Here's how the part is built. I have some questions about the finished solid (model axes, mm). Round coordinates to 2 decimals unless told otherwise and drop trailing zeros. Loops run counter-clockwise (first coordinate to the right, second up) from the corner with the lowest first, then second, coordinate; pieces in that order, holes last. Notation, with made-up numbers: M 85.5,-7.5 L 116.5,-7.5 A9 cw 116.5,9.5 Z; hole C 35.25,14 d6. An arc over 180 degrees is marked long. Use a Markdown table: item, result.
from build123d import *

# Parameters (mm, degrees)
F1_DEPTH = 25.4


# Not quite as in the source:
# - a feature names something its author has since deleted; it is built from what else it names


with BuildPart() as f1:
    # F0 (on Front) → F1 (new body)
    with BuildSketch(Plane.XZ):
        with BuildLine():
            Line((-23.1970027089, 51.8983751535), (-44.2315712571, 16.1199513823))
            Line((-44.2315712571, 16.1199513823), (-28.70137633, 16.1199513823))
            ThreePointArc((-28.70137633, 16.1199513823), (-16.1199513823, 22.0364309456), (-3.5385264346, 16.1199513823))
            Line((-3.5385264346, 16.1199513823), (44.2315712571, 16.1199513823))
            Line((44.2315712571, 16.1199513823), (-23.1970027089, 51.8983751535))
        make_face()
        with BuildLine():
            Line((-28.70137633, 16.1199513823), (-44.2315712571, 16.1199513823))
            Line((-44.2315712571, 16.1199513823), (-44.2315712571, -16.1199513823))
            Line((-44.2315712571, -16.1199513823), (44.2315712571, -16.1199513823))
            Line((44.2315712571, -16.1199513823), (44.2315712571, 16.1199513823))
            Line((44.2315712571, 16.1199513823), (-3.5385264346, 16.1199513823))
            ThreePointArc((-3.5385264346, 16.1199513823), (-0.7516202277, 11.2382926218), (0.215521602, 5.7009579614))
            ThreePointArc((0.215521602, 5.7009579614), (-21.6572860427, -9.6673731932), (-28.70137633, 16.1199513823))
        make_face()
    extrude(amount=F1_DEPTH)


solid = f1.part
1. I need wall thicknesses on probe 1 along X at (y, z) = (-12.25, 6.5); probe 2 along Z at (x, y) = (-27, -21.5); probe 3 along Z at (x, y) = (-23.5, -22.75). Which ranges of each line are inside material? Lowest first, please. Write a range as from..to.
Answer sheet:
| item | result |
|---|---|
| probe 1 | -44.23..-32.44, 0.2..44.23 |
| probe 2 | -16.12..-6.48, 17.89..45.43 |
| probe 3 | -16.12..-8.87, 20.27..51.38 |
2. Imagine slicing it at D-D, the plane x = 22.5. Write out the boundary of the cut face in (y, z), then the cut area to 3 significant figures.
Answer sheet:
| item | result |
|---|---|
| outline | M -25.4,-16.12 L 0,-16.12 L 0,27.65 L -25.4,27.65 Z |
| area | 1,110 mm2 |
3. Imagine slicing it at A-A, the plane y = -20.75. Write out the boundary of the cut face in (x, z).
Answer sheet:
| item | result |
|---|---|
| outline | M -44.23,-16.12 L 44.23,-16.12 L 44.23,16.12 L -23.2,51.9 L -44.23,16.12 Z; hole C -16.12,5.7 d32.67 |
4. Imagine slicing it at C-C, the plane x = -22. Write out the boundary of the cut face in (y, z).
Answer sheet:
| item | result |
|---|---|
| outline | M -25.4,-16.12 L 0,-16.12 L 0,-9.54 L -25.4,-9.54 Z; M -25.4,20.94 L 0,20.94 L 0,51.26 L -25.4,51.26 Z |
5. For pin 1 Ø1.5 at (y, z) = (-6, 43.5) entering from +X; pin 2 Ø4 at (x, y) = (-7, -7) entering from +Z; pin 3 Ø3 at (x, y) = (24, -13) entering from +Z, each with a flat end and sliding along its axis, tell me the tip position at first contact or that it passes through.
Answer sheet:
| item | result |
|---|---|
| pin 1 | x = -5.96 |
| pin 2 | z = 44.37 |
| pin 3 | z = 27.65 |
6. Imagine slicing it at B-B, the plane z = 1. Write out the boundary of the cut face in (x, y).
Answer sheet:
| item | result |
|---|---|
| outline | M -44.23,-25.4 L -31.76,-25.4 L -31.76,0 L -44.23,0 Z; M -0.48,-25.4 L 44.23,-25.4 L 44.23,0 L -0.48,0 Z |
